Input: part model. Units: mm. Frame: model coordinates. A direction names the side the tool comes from. Coordinates: 2 decimals unless noted, no trailing zeros. Loops run counter-clockwise (first coordinate to the right, second up) from the corner with the lowest first, then second, coordinate; pieces in that order, holes last. Notation, with made-up numbers: (-2, 57) -> (12, 57) arc R19 cw to (12, 63) -> close; hole circle Ø1 at (37, 44.5). An arc over 180 degrees is marked (long way). Answer as a JSON object with one key per item and string values.
Autodesk Inventor part; units mm, degrees
ref_plane "YZ Plane" through (0, 0, 0) normal (1, 0, 0) x (0, 1, 0)
ref_plane "XZ Plane" through (0, 0, 0) normal (0, 1, 0) x (-1, 0, 0)
ref_plane "XY Plane" through (0, 0, 0) normal (0, 0, 1) x (1, 0, 0)
sketch "Sketch1" plane through (0, 0, 0) normal (0, 1, 0) x (-1, 0, 0)
  line L0 (0, 0) -> (-28, 0)
  line L1 (-28, 0) -> (-28, -75)
  line L2 (-28, -75) -> (0, -75)
  line L3 (0, -75) -> (0, 0)
  line L4 (-4, -51) -> (-24, -51) construction
  line L5 (-24, -51) -> (-24, -71) construction
  line L6 (-24, -71) -> (-4, -71) construction
  line L7 (-4, -71) -> (-4, -51) construction
  line L8 (-4, -51) -> (-24, -71) construction
  line L9 (-24, -51) -> (-4, -71) construction
  line L10 (-4, -71) -> (-4, -66) construction
  line L11 (-2.5, -71) -> (-2.5, -66)
  line L12 (-5.5, -66) -> (-5.5, -71)
  arc A0 (-5.5, -71) -> (-2.5, -71) centre (-4, -71) ccw
  arc A1 (-2.5, -66) -> (-5.5, -66) centre (-4, -66) ccw
  line L13 (-24, -71) -> (-24, -66) construction
  line L14 (-22.5, -71) -> (-22.5, -66)
  line L15 (-25.5, -66) -> (-25.5, -71)
  arc A2 (-25.5, -71) -> (-22.5, -71) centre (-24, -71) ccw
  arc A3 (-22.5, -66) -> (-25.5, -66) centre (-24, -66) ccw
  line L16 (-4, -51) -> (-4, -46) construction
  line L17 (-2.5, -51) -> (-2.5, -46)
  line L18 (-5.5, -46) -> (-5.5, -51)
  arc A4 (-5.5, -51) -> (-2.5, -51) centre (-4, -51) ccw
  arc A5 (-2.5, -46) -> (-5.5, -46) centre (-4, -46) ccw
  line L19 (-24, -51) -> (-24, -46) construction
  line L20 (-22.5, -51) -> (-22.5, -46)
  line L21 (-25.5, -46) -> (-25.5, -51)
  arc A6 (-25.5, -51) -> (-22.5, -51) centre (-24, -51) ccw
  arc A7 (-22.5, -46) -> (-25.5, -46) centre (-24, -46) ccw
  circle A8 centre (-6.5, -10) radius 1.5
  circle A9 centre (-21.5, -10) radius 1.5
  line L22 (-6.5, -10) -> (-21.5, -10) construction
  point P0 (-14, -61)
  point P1 (-14, -61)
  point P2 (-14, -75)
  point P3 (-4, -68.5)
  point P4 (-24, -68.5)
  point P5 (-4, -48.5)
  point P6 (-24, -48.5)
  point P7 (-14, -10)
  point P8 (-14, 0)
  dimension "d0" = 75
  dimension "d1" = 28
  dimension "d2" = 20
  dimension "d3" = 20
  dimension "d4" = 4
  dimension "d5" = 5
  dimension "d6" = 3
  dimension "d7" = 5
  dimension "d8" = 3
  dimension "d9" = 5
  dimension "d10" = 3
  dimension "d11" = 5
  dimension "d12" = 3
  dimension "d16" = 3
  dimension "d17" = 3
  dimension "d18" = 15
  dimension "d19" = 10
extrude "Extrusion1" add sketch "Sketch1" along normal blind 3 contours L3 L2 L1 L0 | A8 | A9
fillet "Fillet1" radius 3 4 edges at (0, 1.5, 0) (28, 1.5, 0) (0, 1.5, -75) (28, 1.5, -75)
extrude "Extrusion2" cut sketch "Sketch1" along normal through all contours A8 | A9
properties part number "EncoderPCBMount" material "ABS Plastic"
1. Section query A-A (x = 4). Return loops of the section in (y, z).
Reply:
{"outline": "(0, -75) -> (3, -75) -> (3, -72.5) -> (0, -72.5) -> close; (0, -64.5) -> (3, -64.5) -> (3, -52.5) -> (0, -52.5) -> close; (0, -44.5) -> (3, -44.5) -> (3, 0) -> (0, 0) -> close"}
2. Line query: line 1 along X through (y, z) = (1.05, -49.5); line 2 along X through (y, z) = (0.85, -10); line 3 along Z through (x, y) = (21.5, 1.45). Output: solid intervals per line, ascending.
Reply:
{"line 1": "x = 0 to 2.5, 5.5 to 22.5, 25.5 to 28", "line 2": "x = 0 to 5, 8 to 20, 23 to 28", "line 3": "z = -75 to -11.5, -8.5 to 0"}
3. Section query D-D (y = 1.95). Return loops of the section in (x, z), plus the area to 3 significant figures.
Reply:
{"outline": "(0, -72) arc R3 ccw to (3, -75) -> (25, -75) arc R3 ccw to (28, -72) -> (28, -3) arc R3 ccw to (25, 0) -> (3, 0) arc R3 ccw to (0, -3) -> close; hole (2.5, -71) arc R1.5 ccw to (5.5, -71) -> (5.5, -66) arc R1.5 ccw to (2.5, -66) -> close; hole (2.5, -51) arc R1.5 ccw to (5.5, -51) -> (5.5, -46) arc R1.5 ccw to (2.5, -46) -> close; hole circle Ø3 at (6.5, -10); hole circle Ø3 at (21.5, -10); hole (22.5, -71) arc R1.5 ccw to (25.5, -71) -> (25.5, -66) arc R1.5 ccw to (22.5, -66) -> close; hole (22.5, -51) arc R1.5 ccw to (25.5, -51) -> (25.5, -46) arc R1.5 ccw to (22.5, -46) -> close", "area": "1,990 mm2"}
4. Section query B-B (x = 21.5). Return loops of the section in (y, z), plus the area to 3 significant figures.
Reply:
{"outline": "(0, -75) -> (3, -75) -> (3, -11.5) -> (0, -11.5) -> close; (0, -8.5) -> (3, -8.5) -> (3, 0) -> (0, 0) -> close", "area": "216 mm2"}
5. Section query C-C (z = -70). Return loops of the section in (x, y), plus the area to 3 significant figures.
Reply:
{"outline": "(0, 0) -> (2.5, 0) -> (2.5, 3) -> (0, 3) -> close; (5.5, 0) -> (22.5, 0) -> (22.5, 3) -> (5.5, 3) -> close; (25.5, 0) -> (28, 0) -> (28, 3) -> (25.5, 3) -> close", "area": "66.0 mm2"}
6. Access query for faces 1 (the face through (14, 1, 0)), 2 (the face through (22.5, 1, -69)). Directions: +Z, -Z, +X, -X, +Y, -Y. A direction counts if a zero-diameter tool reaches every point of the face in a straight line with its end or side. Return the directions, or none.
Reply:
{"face 1": "+Z, +X, -X, +Y, -Y", "face 2": "+Y, -Y"}
7. Mould query, pull axis X, two halves, no side actions, for faces 3 (the face through (28, 1, -37)), 4 (the face through (22.5, 1, -49)), 5 (the face through (14, 1, -75)). Classes: pulls with the +X half, pulls with the -X half, needs draft (parallel to the pull), parting line crosses it, or undercut.
Reply:
{"face 3": "pulls with the +X half", "face 4": "undercut", "face 5": "needs draft"}
